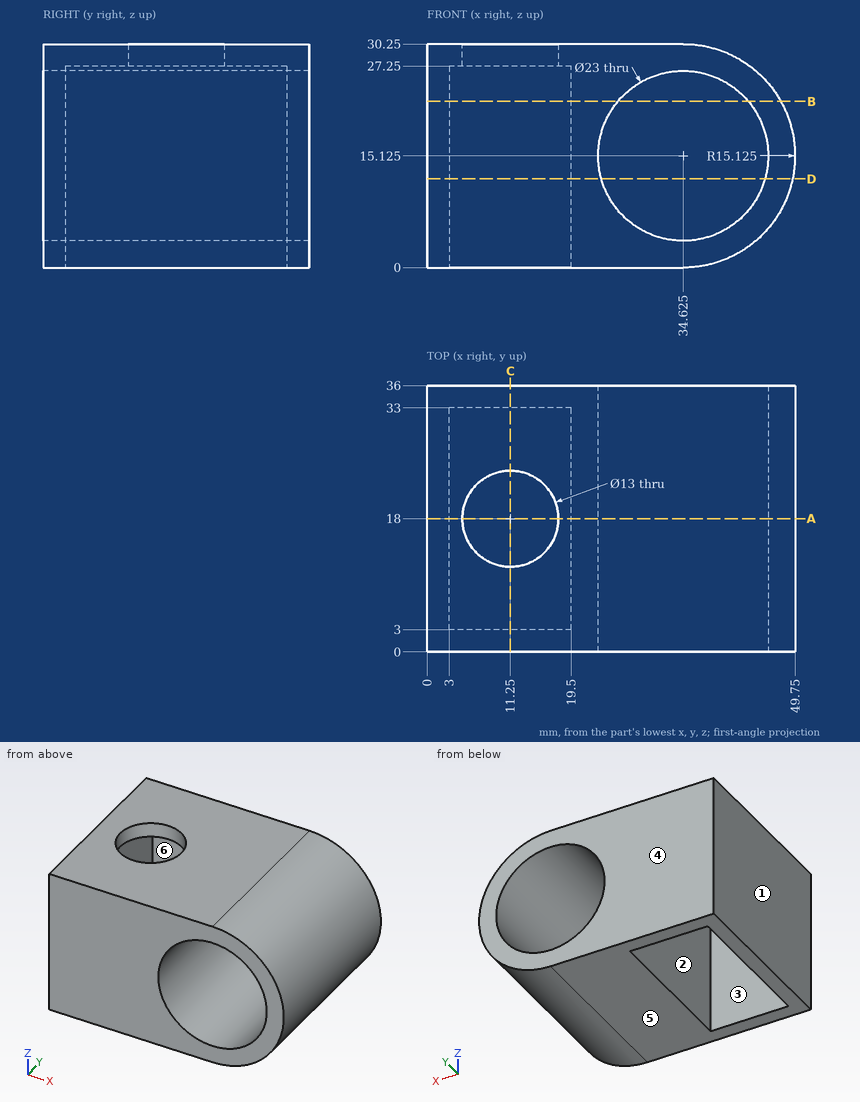
The figure shows three views and two pictorial views of one solid part (mm, origin at its lowest corner). Answer the questions. A direction names the side the tool comes from. Coordinates: 2 decimals unless noted, no trailing zeros. Loops run counter-clockwise (first coordinate to the right, second up) from the corner with the lowest first, then second, coordinate; pieces in that order, holes last. Notation, with made-up numbers: (69, 50) - (77, 50) arc R25 ccw to (77, 69) - close; hole circle Ø2 at (-8.75, -8). An arc over 180 degrees is marked (long way). Write item = value, one per line.
1) Determine the mould class of the marked faces 3, 4, 5 and 6 for opening direction Y: pulls with the +Y half, pulls with the -Y half, needs draft (parallel to the pull), parting line crosses it, or undercut.
Responses:
face_3 = undercut
face_4 = pulls with the +Y half
face_5 = needs draft
face_6 = undercut
2) Section D-D (z = 12) is taken. Determine the outline of the cut face in (x, y), plus the area to 3 significant figures.
Responses:
outline = (0, 0) - (23.56, 0) - (23.56, 36) - (0, 36) - close; (45.69, 0) - (49.42, 0) - (49.42, 36) - (45.69, 36) - close; hole (3, 3) - (19.5, 3) - (19.5, 33) - (3, 33) - close
area = 487 mm^2
3) Section B-B (z = 22.5) is taken. Determine the outline of the cut face in (x, y), plus the area to 3 significant figures.
Responses:
outline = (0, 0) - (25.8, 0) - (25.8, 36) - (0, 36) - close; (43.45, 0) - (47.83, 0) - (47.83, 36) - (43.45, 36) - close; hole (3, 3) - (19.5, 3) - (19.5, 33) - (3, 33) - close
area = 592 mm^2
4) Which of the six approach directions +Z, -Z, +X, -X, +Y, -Y give full straight-line access (tool end or side, diameter ignored) to the marked faces 1 and 2?
Responses:
face_1 = +Z, -Z, -X, +Y, -Y
face_2 = -Z
5) Section A-A (y = 18) is taken. Determine the outline of the cut face in (x, z) (3 decimals), plus the area to 3 significant figures.
Responses:
outline = (0, 0) - (3, 0) - (3, 27.25) - (4.75, 27.25) - (4.75, 30.25) - (0, 30.25) - close; (17.75, 27.25) - (19.5, 27.25) - (19.5, 0) - (34.625, 0) arc R15.125 ccw to (34.625, 30.25) - (17.75, 30.25) - close; hole circle Ø23 at (34.625, 15.125)
area = 503 mm^2
6) Find the intervals of material crossed by line 1 along Y through (x, z) = (18, 24); line 2 along Y through (x, z) = (11.25, 28.8); line 3 along X through (y, z) = (4, 17.5), in increasing order.
Responses:
line_1 = 0 to 3, 33 to 36
line_2 = 0 to 11.5, 24.5 to 36
line_3 = 0 to 3, 19.5 to 23.37, 45.88 to 49.56
7) Each of these flat-tipped pins is pushed along its axis until it touches: P1, Ø5, axis at y = 31, z = 25.5, coming from the +X side; P2, Ø10, axis at y = 24.5, z = 9.5, coming from the +X side. Where does it stop, or does it pass through?
Responses:
P1 = 47.54
P2 = 49.74
8) Section C-C (x = 11.25) is taken. Determine the outline of the cut face in (y, z).
Responses:
outline = (0, 0) - (3, 0) - (3, 27.25) - (11.5, 27.25) - (11.5, 30.25) - (0, 30.25) - close; (24.5, 27.25) - (33, 27.25) - (33, 0) - (36, 0) - (36, 30.25) - (24.5, 30.25) - close
